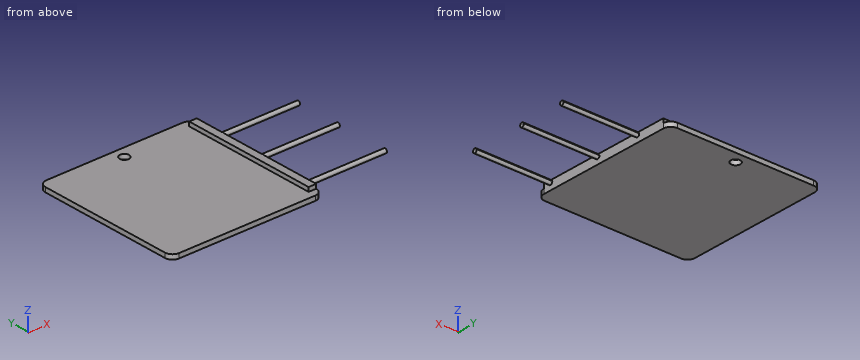
from build123d import *

# Parameters (mm, degrees)
F1_DEPTH = 1.5494
F2_R     = 1.5875
F3_DEPTH = 25.4
F5_W     = 2.54
F5_H     = 45.72
F6_DEPTH = 1.397
F7_DEPTH = 25.4


# Not quite as in the source:
# - a feature names something its author has since deleted; it is built from what else it names


with BuildPart() as f1:
    # F0 (on Top) → F1 (new body)
    with BuildSketch(Plane.XY):
        with BuildLine():
            ThreePointArc((0, 2.54), (0.7439487758, 0.7439487758), (2.54, 0))
            Line((2.54, 0), (48.26, 0))
            ThreePointArc((48.26, 0), (50.0560512242, 0.7439487758), (50.8, 2.54))
            Line((50.8, 2.54), (50.8, 48.26))
            ThreePointArc((50.8, 48.26), (50.0560512242, 50.0560512242), (48.26, 50.8))
            Line((48.26, 50.8), (2.54, 50.8))
            ThreePointArc((2.54, 50.8), (0.7439487758, 50.0560512242), (0, 48.26))
            Line((0, 48.26), (0, 2.54))
        make_face()
    extrude(amount=F1_DEPTH)

    # F2 (on face) → F3 (cut)
    with BuildSketch(Plane.XY.offset(1.5494)):
        with Locations((25.4, 46.99)):
            Circle(F2_R)
    extrude(amount=-F3_DEPTH, mode=Mode.SUBTRACT)

    # F5 (on face) → F6 (join)
    with BuildSketch(Plane.XY.offset(1.5494)):
        with Locations((49.53, 25.4)):
            Rectangle(F5_W, F5_H)
    extrude(amount=F6_DEPTH)

    # F4 (on face) → F7 (join)
    with BuildSketch(Plane.YZ.offset(50.8)):
        with BuildLine():
            ThreePointArc((5.0799999892, 1.5494), (5.5739140828, 1.7539859095), (5.7785, 2.2479))
            ThreePointArc((5.7785, 2.2479), (4.5860859172, 2.7418140905), (5.0799999892, 1.5494))
        make_face()
        with BuildLine():
            ThreePointArc((23.8125, 2.2479), (22.6200859133, 2.7418140867), (23.114, 1.5494))
            ThreePointArc((23.114, 1.5494), (23.6079140867, 1.7539859133), (23.8125, 2.2479))
        make_face()
        with BuildLine():
            ThreePointArc((39.0525, 2.2479), (37.8600859133, 2.7418140867), (38.354, 1.5494))
            ThreePointArc((38.354, 1.5494), (38.8479140867, 1.7539859133), (39.0525, 2.2479))
        make_face()
    extrude(amount=F7_DEPTH)


solid = f1.part
Could you check a few things on this model? Use its own coordinates, in mm. Coordinates: 2 decimals unless noted, no trailing zeros. Loops run counter-clockwise (first coordinate to the right, second up) from the corner with the lowest first, then second, coordinate; pieces in that order, holes last.
1. Imagine slicing it at D-D (y = 18). Please give me the cut outline in (x, z), and give its area (3 significant figures).
2. Imagine slicing it at C-C (x = 53). Please give me the cut outline in (y, z).
3. For P1, Ø1.1, axis at x = 49.5, z = 2, coming from the -Y side; P2, Ø1, axis at x = 28, y = 20, coming from the +Z side; P3, Ø3.5, axis at x = 25.4, y = 46.99, coming from the -Z side; P4, Ø1.5, axis at x = 49, z = 2, coming from the +Y side, each with a flat end and sliding along its axis, tell me the tip position at first contact or that it passes through.
4. Imagine slicing it at A-A (x = 25.4). Please give me the cut outline in (y, z).
5. I need wall thicknesses on L1, parallel to Y at x = 54.5, z = 2.3; L2, parallel to Y at x = 25.4, z = 0.8; L3, parallel to Y at x = 72, z = 2.55. Which ranges of each line are inside material? Lowest first, please.
6. Imagine slicing it at B-B (z = 0.5). Please give me the cut outline in (x, y) (1 decimal), and give its area (3 significant figures).
Computed values:
1. outline: (0, 0) - (50.8, 0) - (50.8, 2.95) - (48.26, 2.95) - (48.26, 1.55) - (0, 1.55) - close
1. area: 82.3 mm2
2. outline: circle Ø1.4 at (5.08, 2.25); circle Ø1.4 at (23.11, 2.25); circle Ø1.4 at (38.35, 2.25)
3. P1: stops at y = 0.17
3. P2: stops at z = 1.55
3. P3: stops at z = 0
3. P4: stops at y = 50.8
4. outline: (0, 0) - (45.4, 0) - (45.4, 1.55) - (0, 1.55) - close; (48.58, 0) - (50.8, 0) - (50.8, 1.55) - (48.58, 1.55) - close
5. L1: y = 4.38 to 5.78, 22.42 to 23.81, 37.66 to 39.05
5. L2: y = 0 to 45.4, 48.58 to 50.8
5. L3: y = 4.45 to 5.71, 22.48 to 23.74, 37.72 to 38.98
6. outline: (0, 2.5) arc R2.5 ccw to (2.5, 0) - (48.3, 0) arc R2.5 ccw to (50.8, 2.5) - (50.8, 48.3) arc R2.5 ccw to (48.3, 50.8) - (2.5, 50.8) arc R2.5 ccw to (0, 48.3) - close; hole circle Ø3.2 at (25.4, 47)
6. area: 2,570 mm2
